Input: part model. Units: mm. Frame: model coordinates. A direction names the side the tool comes from. Coordinates: 2 decimals unless noted, no trailing zeros. Loops run counter-clockwise (first coordinate to the right, second up) from the corner with the lowest first, then second, coordinate; pieces in that order, holes last. Notation, with made-up numbers: (-12, 60.5) - (13, 60.5) arc R19 ccw to (13, 68.5) - close; hole circle Ø4 at (46, 18). An arc over 180 degrees is marked (long way). Use one line per item in the form item = value.
from build123d import *

# Parameters (mm, degrees)
SKETCH1_W           = 15
SKETCH1_H           = 10.5
BOSS_EXTRUDE1_DEPTH = 1.6
SKETCH2_W           = 10.3
SKETCH2_H           = 6.5
CUT_EXTRUDE1_DEPTH  = 1.5
SKETCH3_W           = 10.2
SKETCH3_H           = 6.4
BOSS_EXTRUDE2_DEPTH = 4.1
CUT_EXTRUDE4_DEPTH  = 6.4
SKETCH8_W           = 13.2
SKETCH8_H           = 8.4
BOSS_EXTRUDE5_DEPTH = 8.1
SKETCH9_W           = 0.6
SKETCH9_H           = 6.1
CUT_EXTRUDE30_DEPTH = 8.4
SKETCH10_W          = 0.6
SKETCH10_H          = 2
BOSS_EXTRUDE7_DEPTH = 0.4
LPATTERN3_COUNT     = 2
LPATTERN3_PITCH     = 8.8
SKETCH12_W          = 1.719741978
SKETCH12_H          = 6.045276093
BOSS_EXTRUDE8_DEPTH = 1.1
CUT_EXTRUDE42_DEPTH = 1.1


with BuildPart() as part:
    # Sketch1 → Boss-Extrude1 (new body)
    with BuildSketch(Plane(origin=(0, 0, 0), x_dir=(1, 0, 0), z_dir=(0, 1, 0))):
        Rectangle(SKETCH1_W, SKETCH1_H)
    extrude(amount=BOSS_EXTRUDE1_DEPTH)

    # Sketch2 → Cut-Extrude1 (cut)
    with BuildSketch(Plane(origin=(0, 1.6, 0), x_dir=(1, 0, 0), z_dir=(0, 1, 0))):
        Rectangle(SKETCH2_W, SKETCH2_H)
    extrude(amount=-CUT_EXTRUDE1_DEPTH, mode=Mode.SUBTRACT)

    # Sketch3 → Boss-Extrude2 (add)
    with BuildSketch(Plane(origin=(0, 0.1, 0), x_dir=(1, 0, 0), z_dir=(0, 1, 0))):
        Rectangle(SKETCH3_W, SKETCH3_H)
    extrude(amount=BOSS_EXTRUDE2_DEPTH)

    # Sketch4 → Cut-Extrude4 (cut)
    with BuildSketch(Plane.XY.offset(3.2)):
        Polygon((-5.1, 4.2), (-5.1, 1.33831827), (-3.296595892, 4.2), align=None)
        with BuildLine():
            Line((5.1, 4.2), (-3.296595892, 4.2))
            ThreePointArc((-3.296595892, 4.2), (0.730166495, 2.35961781), (5.1, 1.648016048))
            Line((5.1, 1.648016048), (5.1, 4.2))
        make_face()
    extrude(amount=-CUT_EXTRUDE4_DEPTH, mode=Mode.SUBTRACT)



with BuildPart() as body_2:
    # Sketch8 → Boss-Extrude5 (new body)
    with BuildSketch(Plane(origin=(0, 0, 0), x_dir=(-1, 0, 0), z_dir=(0, -1, 0))):
        Rectangle(SKETCH8_W, SKETCH8_H)
    extrude(amount=BOSS_EXTRUDE5_DEPTH)

    # Sketch9 → Cut-Extrude30 (cut)
    with BuildSketch(Plane.XY.offset(4.2)):
        with Locations((-6.3, -3.05)):
            Rectangle(SKETCH9_W, SKETCH9_H)
        with Locations((6.3, -3.05)):
            Rectangle(SKETCH9_W, SKETCH9_H)
    extrude(amount=-CUT_EXTRUDE30_DEPTH, mode=Mode.SUBTRACT)


with BuildPart() as part_1:
    add(part.part)

    add(body_2.part)  # Boss-Extrude7 merges body 2
    # Sketch10 → Boss-Extrude7 (add)
    with BuildSketch(Plane(origin=(0, 0, -4.2), x_dir=(-1, 0, 0), z_dir=(0, 0, -1))):
        with Locations((-5.7, -1)):
            Rectangle(SKETCH10_W, SKETCH10_H)
        with Locations((5.7, -1)):
            Rectangle(SKETCH10_W, SKETCH10_H)
    boss_extrude7 = extrude(amount=BOSS_EXTRUDE7_DEPTH)

    # LPattern3: Boss-Extrude7 ×2
    with Locations(*[(0, 0, i * LPATTERN3_PITCH) for i in range(1, LPATTERN3_COUNT)]):
        add(boss_extrude7)

    # Sketch12 → Boss-Extrude8 (add)
    with BuildSketch(Plane.ZY.offset(6)):
        with Locations((0, -3.045413524)):
            Rectangle(SKETCH12_W, SKETCH12_H)
    extrude(amount=BOSS_EXTRUDE8_DEPTH)

    # Sketch14 → Cut-Extrude42 (cut)
    with BuildSketch(Plane(origin=(0, 0, -0.859870989), x_dir=(-1, 0, 0), z_dir=(0, 0, -1))):
        Polygon((7.1, -0.022775477), (6.422538679, -0.022775477), (7.012651067, -3.06805157), (6.422765107, -6.06805157), (7.1, -6.06805157), align=None)
    extrude(amount=-CUT_EXTRUDE42_DEPTH, mode=Mode.SUBTRACT)


solid = part_1.part
Q1. Pull-direction query (Y, two-part tool) for faces 4 (the flat face through (-6.4, -3.1, -0.86)), 5 (the cylindrical face through (0.67, 2.38, 0.04)), 6 (the flat face through (-6.6, -7, 0)); classes: pulls with the +Y half, pulls with the -Y half, needs draft (parallel to the pull), parting line crosses it, or undercut.
Check values:
face_4 = undercut
face_5 = pulls with the +Y half
face_6 = needs draft
Q2. Cut plane C-C, the plane x = -2.5. Return loops of the section in (y, z), then the cut area to 3 significant figures.
Check values:
outline = (-8.1, -4.2) - (0, -4.2) - (0, -5.25) - (1.6, -5.25) - (1.6, -3.25) - (0.1, -3.25) - (0.1, -3.2) - (3.73, -3.2) - (3.73, 3.2) - (0.1, 3.2) - (0.1, 3.25) - (1.6, 3.25) - (1.6, 5.25) - (0, 5.25) - (0, 4.2) - (-8.1, 4.2) - close
area = 98.3 mm²
Q3. Cut plane D-D, the plane z = 2.25. Return loops of the section in (x, y).
Check values:
outline = (-7.5, 0) - (-6, 0) - (-6, -6.1) - (-6.6, -6.1) - (-6.6, -8.1) - (6.6, -8.1) - (6.6, -6.1) - (6, -6.1) - (6, 0) - (7.5, 0) - (7.5, 1.6) - (5.15, 1.6) - (5.15, 0.1) - (5.1, 0.1) - (5.1, 1.65) arc R16.62 cw to (-3.3, 4.2) - (-5.1, 1.34) - (-5.1, 0.1) - (-5.15, 0.1) - (-5.15, 1.6) - (-7.5, 1.6) - close
Q4. Ray query, line 1 along Y through (x, z) = (-6.25, -3.5); line 2 along X through (y, z) = (-7, -1); line 3 along Z through (x, y) = (2.25, -1.75). Return the intervals inside material, ascending. Write a range as [from, to].
Check values:
line_1 = [-8.1, -6.1], [0, 1.6]
line_2 = [-6.6, 6.6]
line_3 = [-4.2, 4.2]
Q5. Cut plane A-A, the plane z = -4. Return loops of the section in (x, y), then the cut area to 3 significant figures.
Check values:
outline = (-7.5, 0) - (-6, 0) - (-6, -6.1) - (-6.6, -6.1) - (-6.6, -8.1) - (6.6, -8.1) - (6.6, -6.1) - (6, -6.1) - (6, 0) - (7.5, 0) - (7.5, 1.6) - (-7.5, 1.6) - close
area = 124 mm²
Q6. First-contact query: P1, Ø2, axis at y = -4.5, z = 2, coming from the -X side; P2, Ø0.5, axis at x = -6, y = -1.5, coming from the -Z side; P3, Ø0.5, axis at x = -6.5, y = -4, coming from the -Z side. Flat tips, straight axial feed; report the tip coordinate or a pass-through.
Check values:
P1 = -6
P2 = -4.6
P3 = -0.86
Q7. Set-up query: faces 1 (the flat face through (7.5, 1, 0)), 2 (the flat face through (-6.5, -3.1, 0.86)), 3 (the flat face through (-6.713, -1.524, -0.318)). Return all of +Z, -Z, +X, -X, +Y, -Y with unobstructed straight access to the full face (end or side cutting, diameter ignored); none if empty.
Check values:
face_1 = +Z, -Z, +X, +Y, -Y
face_2 = +Z, -X
face_3 = -Z, -X
Q8. Cut plane B-B, the plane y = -5. Return loops of the section in (x, z), then the cut area to 3 significant figures.
Check values:
outline = (-7.1, 0.24) - (-6.63, 0.24) - (-6.63, -0.86) - (-6, -0.86) - (-6, -4.2) - (6, -4.2) - (6, 4.2) - (-6, 4.2) - (-6, 0.86) - (-7.1, 0.86) - close
area = 102 mm²
